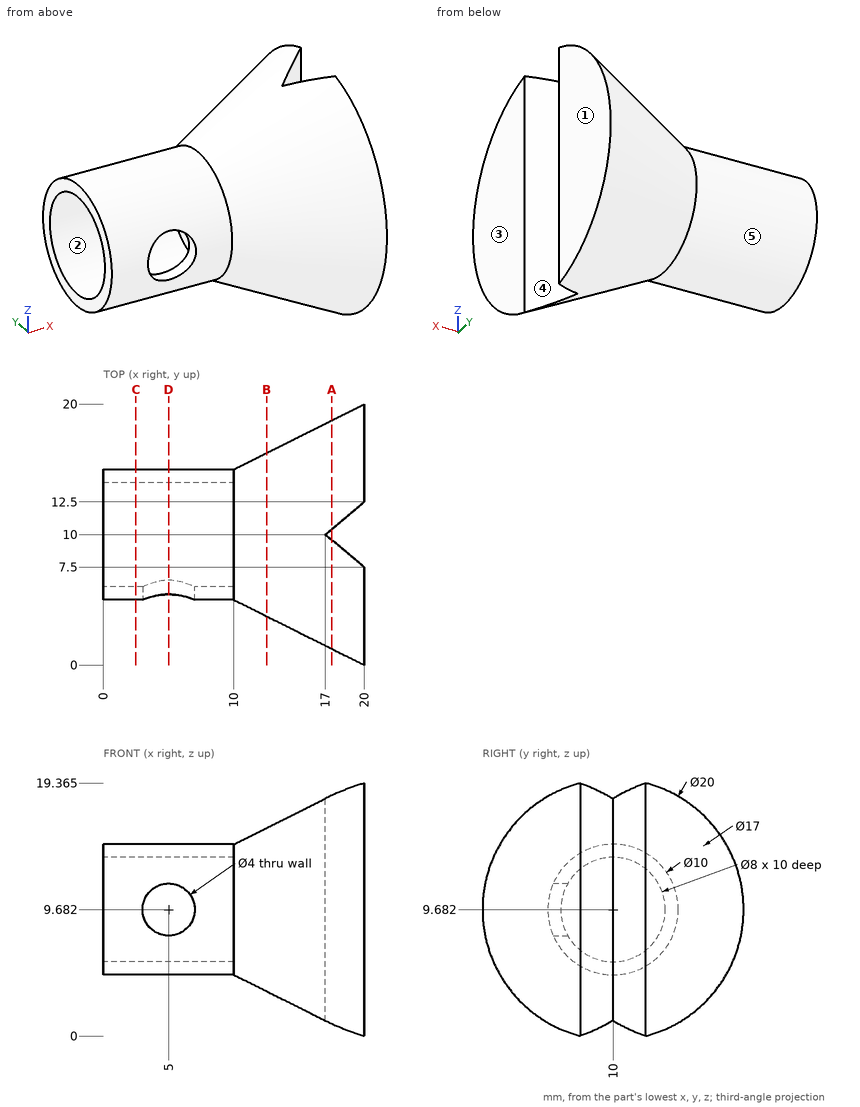
Geometry check sheet. Reference: drawing and pictorial views, mm from the part's lowest x, y, z. A direction names the side the tool comes from. Give positions to 0.01 mm unless a question says otherwise; leave off trailing zeros. Loops run counter-clockwise (first coordinate to the right, second up) from the corner with the lowest first, then second, coordinate; pieces in that order, holes last. Notation, with made-up numbers: M 68.25,72.25 L 114.25,72.25 A24 cw 114.25,89.25 Z; hole C 81,47.5 d6. An arc over 180 degrees is marked long. One line per question, with ' | ' between items.
Item 1: Section check D-D, the plane x = 5. Record the cut outline in (y, z) (1 decimal).
Completed:
outline: M 5.4,7.7 A5 ccw long 5.4,11.7 L 6.5,11.7 A4 cw long 6.5,7.7 Z
Item 2: Draft check along Y on the marked faces 3, 4 and 5. Enter one of: +Y half, -Y half, draft (parallel to the pull), parting line (faces both ways), or undercut.
Completed:
face 3: draft | face 4: undercut | face 5: parting line
Item 3: Depth check by flat-ended pin: P1, Ø1, axis at x = 14.5, y = 4, coming from the +Z side; P2, Ø4, axis at x = 3.5, z = 5, coming from the -Y side; P3, Ø1.5, axis at x = 9.5, y = 17, coming from the -Z side; P4, Ø5, axis at x = 16, z = 8, coming from the +Y side. Enter the tip coordinate at first touch or a pass-through.
Completed:
P1: stops at z = 14.52 | P2: stops at y = 5.78 | P3: passes through | P4: stops at y = 19.15
Item 4: Thickness scan on line 1 (Z direction, x = 6.5, y = 10); line 2 (Y direction, x = 18.5, z = 13.75); line 3 (Y direction, x = 8.25, z = 9.25). Record the ranges inside material, lowest first. Write a range as [from, to].
Completed:
line 1: z = [4.68, 5.68], [13.68, 14.68] | line 2: y = [1.69, 8.75], [11.25, 18.31] | line 3: y = [5.02, 6.02], [13.98, 14.98]
Item 5: Section check A-A, the plane x = 17.5. Record the cut outline in (y, z).
Completed:
outline: M 9.58,0.94 L 9.58,18.42 A8.75 ccw Z; M 10.42,0.94 A8.75 ccw 10.42,18.42 Z
Item 6: Section check B-B, the plane x = 12.5. Record the cut outline in (y, z), plus the area to 3 significant figures.
Completed:
outline: C 10,9.68 d12.5 | area: 123 mm^2
Item 7: Section check C-C, the plane x = 2.5. Record the cut outline in (y, z).
Completed:
outline: C 10,9.68 d10; hole C 10,9.68 d8
Item 8: Tool access check on the marked faces 1 and 2. Record the directions out of +Z, -Z, +X, -X, +Y, -Y that give a thin tool (end or side, any length) a straight path to the whole face; none if there is none.
Completed:
face 1: +Z, -Z, +X, +Y, -Y | face 2: -X
